Print and shaded views of the part. All mm, measured from the part's lowest x, y and z. Coordinates: 2 decimals unless noted, no trailing zeros. One line per item, written item: value. Start each with the question number.
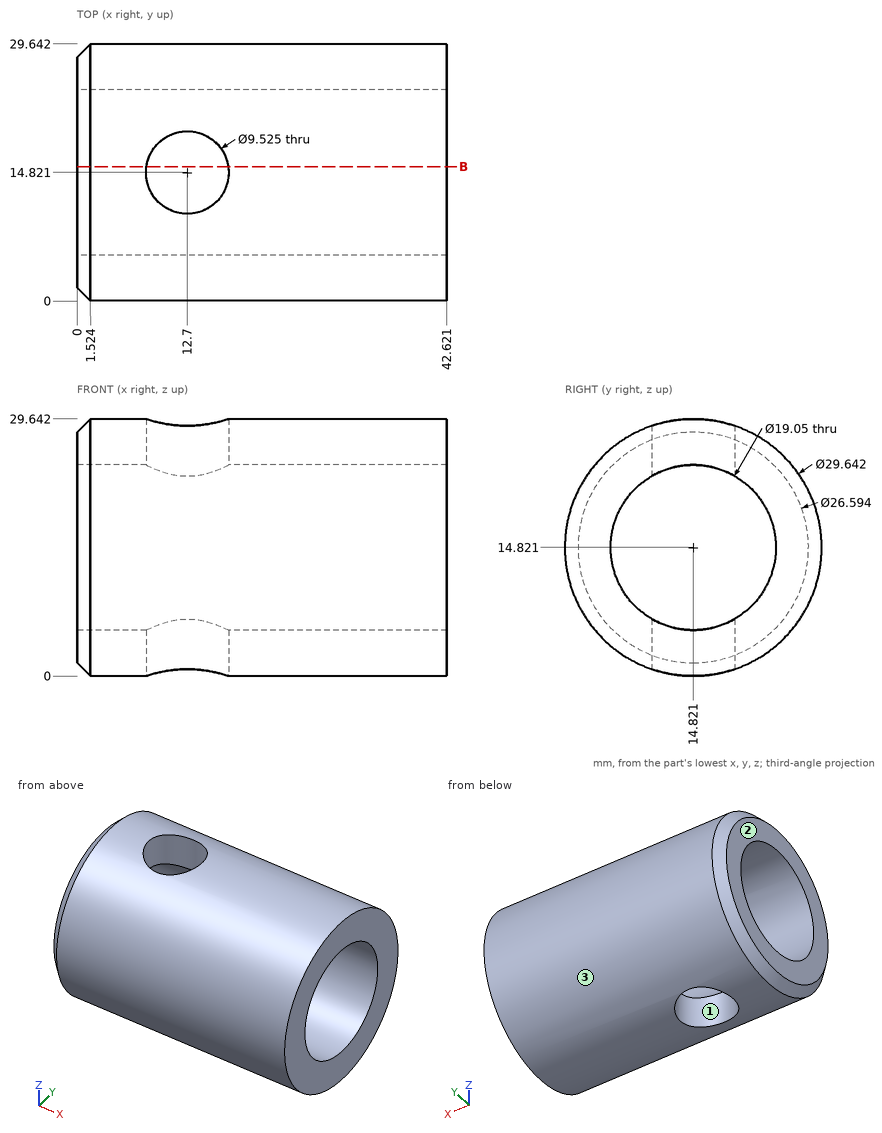
1) Pull direction Y, two halves, no side cores. Call the marked faces 1, 2 and 3: +Y half, -Y half, draft (parallel to the pull), parting line (faces both ways), or undercut.
2) Pin check, flat tips, straight feed: pin 1 Ø10 at (y, z) = (6.5, 11) entering from -X; pin 2 Ø3 at (x, z) = (20, 23) entering from +Y; pin 3 Ø5.5 at (x, y) = (12.7, 14.82) entering from -Z; pin 4 Ø6 at (x, y) = (12, 3) entering from +Z. Stop position of each tip, or through.
3) Probe line 1 (Y direction, x = 6.5, z = 15); line 2 (Y direction, x = 12.7, z = 27.25) (1 decimal); line 3 (Z direction, x = 39, y = 10.5). List the from-to ranges inside material, lowest first. Write a range as from..to.
4) Slice it at B-B (y = 15.5). State how many separate pieces and enclosed holes the cut face has, then the cut area to 3 significant figures.
Check sheet entries:
1. face 1: undercut
1. face 2: draft
1. face 3: parting line
2. pin 1: stops at x = 0
2. pin 2: stops at y = 28.05
2. pin 3: passes through
2. pin 4: stops at z = 26.73
3. line 1: y = 0..5.3, 24.34..29.64
3. line 2: y = 6.7..10.1, 19.6..22.9
3. line 3: z = 0.64..6.33, 23.31..29
4. separate pieces: 4
4. enclosed holes: 0
4. area: 350 mm^2
